Geometry check sheet. Reference: drawing and pictorial views, mm from the part's lowest x, y, z. A direction names the side the tool comes from. Give positions to 0.01 mm unless a question says otherwise; leave off trailing zeros. Loops run counter-clockwise (first coordinate to the right, second up) from the corner with the lowest first, then second, coordinate; pieces in that order, holes last. Notation, with made-up numbers: (-30.5, 76.25) -> (19.5, 76.25) arc R25 cw to (19.5, 94.25) -> close; hole circle Ø6 at (-23.75, -22). An arc over 180 degrees is marked (long way). Answer in a Markdown table with one row per item. Add a question column.
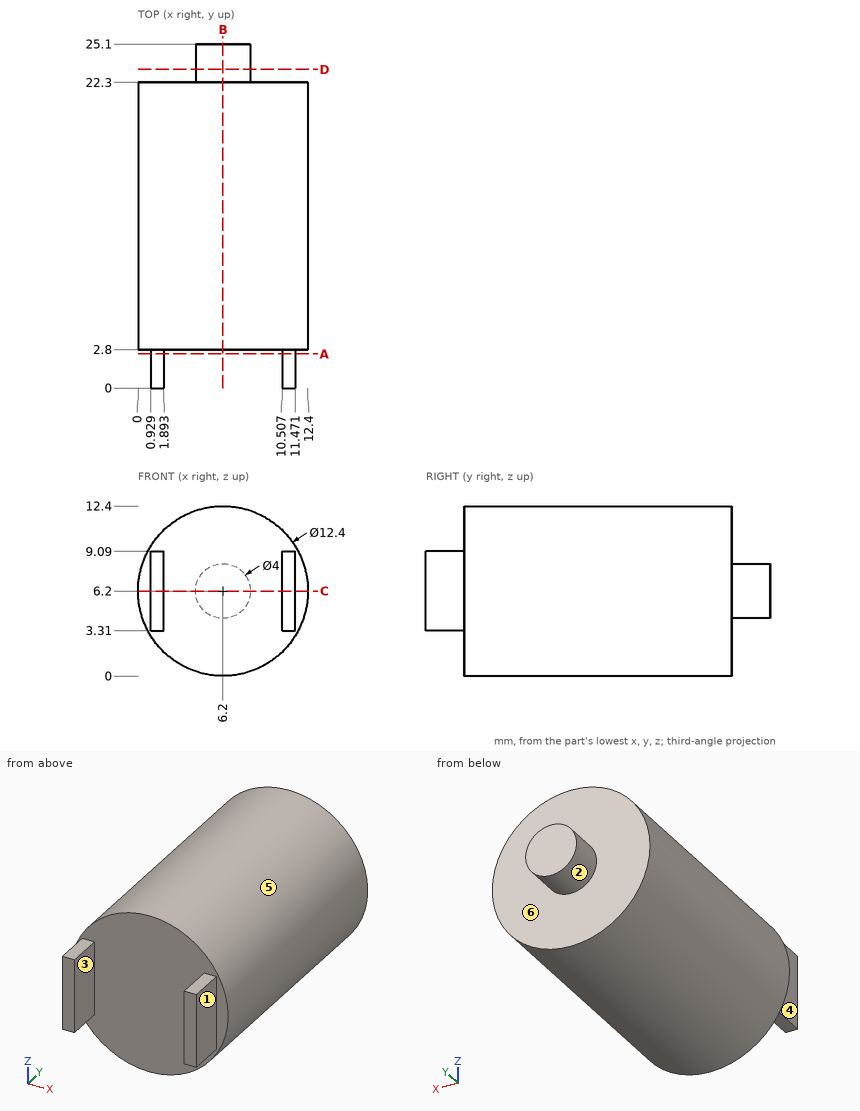
1. Sectioned sample at B-B (x = 6.2). Enter the section's corners in (y, z).
2. Sectioned sample at A-A (y = 2.5). Enter the section's corners in (x, z).
3. Release check for a two-part mould opening along X. For the marked faces 1, 2 and 3 record: released by +X, released by -X, zero draft, split by the parting line, or undercut.
4. Sectioned sample at C-C (z = 6.2). Enter the section's corners in (x, y), plus the area to 3 significant figures.
5. Sectioned sample at D-D (y = 23.25). Enter the section's corners in (x, z), plus the area to 3 significant figures.
6. Material ranges on L1, parallel to Y at x = 2.25, z = 10.5; L2, parallel to Y at x = 6.5, z = 5.25; L3, parallel to Z at x = 6.75, y = 9 (1 decimal), recorded low to high. Write a range as from..to.
7. Gauge pin test, flat ends, axial feed: pin 1 Ø0.8 at (y, z) = (1, 5) entering from +X; pin 2 Ø1.5 at (x, z) = (3, 6.5) entering from -Y; pin 3 Ø1.4 at (y, z) = (1.5, 6) entering from -X. Record the tip position at first contact, or that the pin passes through.
8. Access from +Z, -Z, +X, -X, +Y, -Y to the whole of each face (thin tool, end or side, straight path). Record for the marked faces 4, 5 and 6.
Response:
| question | item | result |
|---|---|---|
| 1 | outline | (2.8, 0) -> (22.3, 0) -> (22.3, 4.2) -> (25.1, 4.2) -> (25.1, 8.2) -> (22.3, 8.2) -> (22.3, 12.4) -> (2.8, 12.4) -> close |
| 2 | outline | (0.93, 3.31) -> (1.89, 3.31) -> (1.89, 9.09) -> (0.93, 9.09) -> close; (10.51, 3.31) -> (11.47, 3.31) -> (11.47, 9.09) -> (10.51, 9.09) -> close |
| 3 | face 1 | released by +X |
| 3 | face 2 | split by the parting line |
| 3 | face 3 | undercut |
| 4 | outline | (0, 2.8) -> (0.93, 2.8) -> (0.93, 0) -> (1.89, 0) -> (1.89, 2.8) -> (10.51, 2.8) -> (10.51, 0) -> (11.47, 0) -> (11.47, 2.8) -> (12.4, 2.8) -> (12.4, 22.3) -> (8.2, 22.3) -> (8.2, 25.1) -> (4.2, 25.1) -> (4.2, 22.3) -> (0, 22.3) -> close |
| 4 | area | 258 mm2 |
| 5 | outline | circle Ø4 at (6.2, 6.2) |
| 5 | area | 12.6 mm2 |
| 6 | L1 | y = 2.8..22.3 |
| 6 | L2 | y = 2.8..25.1 |
| 6 | L3 | z = 0..12.4 |
| 7 | pin 1 | stops at x = 11.47 |
| 7 | pin 2 | stops at y = 2.8 |
| 7 | pin 3 | stops at x = 0.93 |
| 8 | face 4 | +Z, -Z, -X, -Y |
| 8 | face 5 | +Y, -Y |
| 8 | face 6 | +Y |
